Part print with two shaded views. Sizes in mm from the minimum x, y, z corner. A direction names the side the tool comes from. Coordinates: 2 decimals unless noted, no trailing zeros. Loops run counter-clockwise (first coordinate to the right, second up) from the corner with the lowest first, then second, coordinate; pieces in that order, holes last. Notation, with made-up numbers: (70, 60.25) -> (115, 60.25) arc R18 cw to (115, 87.25) -> close; hole circle Ø3 at (-0.5, 3). An arc over 180 degrees is marked (long way). Answer as a JSON object with one key per item and string values. Group by question number.
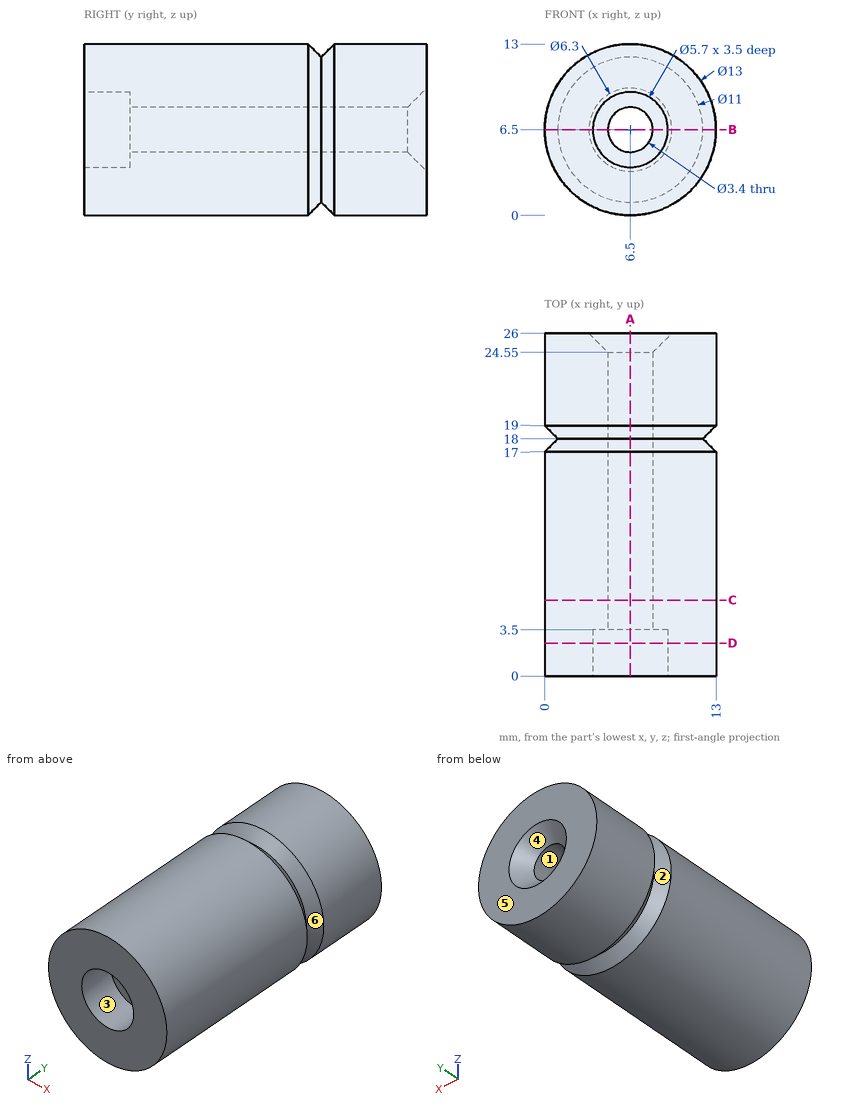
Item 1: 3-axis set-ups, long thin cutter, end or side, ignore diameter. For the marked faces 1, 2 and 3: which of +Z, -Z, +X, -X, +Y, -Y reach the whole face in a straight line?
Item 2: Band-saw the part on A-A, the plane x = 6.5. List the corners of the cut face in (y, z), and give its area (3 significant figures).
Item 3: Pull direction Z, two halves, no side cores. Call the marked faces 4, 5 and 6: +Z half, -Z half, draft (parallel to the pull), parting line (faces both ways), or undercut.
Item 4: Drill centre lines: L1, parallel to X at y = 14.25, z = 6.5; L2, parallel to X at y = 2.4, z = 6.5; L3, parallel to Y at x = 0.5, z = 7.5. Where is each one in solid material? Low to high.
Item 5: Band-saw the part on D-D, the plane y = 2.5. List the corners of the cut face in (x, z), and give its area (3 significant figures).
Item 6: Band-saw the part on B-B, the plane z = 6.5. List the corners of the cut face in (x, y), and give its area (3 significant figures).
Item 7: Flat gauge pins, fed straight in: P1, Ø1.5, axis at x = 10, z = 2.5, coming from the -Y side; P2, Ø3, axis at x = 9, y = 9.5, coming from the -Z side; P3, Ø6, axis at y = 23, z = 10, coming from the -X side; P4, Ø2, axis at x = 9, y = 13, coming from the -Z side. Where does each tip first touch, or does it go through?
Item 8: Band-saw the part on C-C, the plane y = 5.75. List the corners of the cut face in (x, z).
Reply:
{
 "1": {"face 1": "+Y, -Y", "face 2": "none", "face 3": "-Y"},
 "2": {"outline": "(0, 0) -> (17, 0) -> (18, 1) -> (19, 0) -> (26, 0) -> (26, 3.35) -> (24.55, 4.8) -> (3.5, 4.8) -> (3.5, 3.65) -> (0, 3.65) -> close; (0, 9.35) -> (3.5, 9.35) -> (3.5, 8.2) -> (24.55, 8.2) -> (26, 9.65) -> (26, 13) -> (19, 13) -> (18, 12) -> (17, 13) -> (0, 13) -> close", "area": "237 mm²"},
 "3": {"face 4": "undercut", "face 5": "draft", "face 6": "parting line"},
 "4": {"L1": "0 to 4.8, 8.2 to 13", "L2": "0 to 3.65, 9.35 to 13", "L3": "0 to 17.42, 18.58 to 26"},
 "5": {"outline": "circle Ø13 at (6.5, 6.5); hole circle Ø5.7 at (6.5, 6.5)", "area": "107 mm²"},
 "6": {"outline": "(0, 0) -> (3.65, 0) -> (3.65, 3.5) -> (4.8, 3.5) -> (4.8, 24.55) -> (3.35, 26) -> (0, 26) -> (0, 19) -> (1, 18) -> (0, 17) -> close; (8.2, 3.5) -> (9.35, 3.5) -> (9.35, 0) -> (13, 0) -> (13, 17) -> (12, 18) -> (13, 19) -> (13, 26) -> (9.65, 26) -> (8.2, 24.55) -> close", "area": "237 mm²"},
 "7": {"P1": "y = 0", "P2": "z = 0.08", "P3": "x = 0.02", "P4": "z = 0.18"},
 "8": {"outline": "circle Ø13 at (6.5, 6.5); hole circle Ø3.4 at (6.5, 6.5)"}
}
